The model under review builds one solid part; all positions refer to its coordinate system, in mm. A direction names the side the tool comes from. Round coordinates to 2 decimals unless told otherwise and drop trailing zeros. Order: outer loops, then holes, each group sorted by start corner. A loop starts at its lowest first (then second) coordinate and runs counter-clockwise, first axis right, second up. Notation, with made-up numbers: M -18.75,-24 L 0.25,-24 A23 ccw 0.25,-3 Z; hole C 28,84.25 d3. An arc over 180 degrees is marked long. One line per item, written item: value. Start each with the question number.
from build123d import *

# Parameters (mm, degrees)
SKETCH3_R          = 11
SKETCH3_R_2        = 10.2
CUT_EXTRUDE1_REACH = 197.895
SKETCH4_R          = 3.3
SKETCH5_R          = 3.3
CUT_EXTRUDE2_DEPTH = 196.894862351
CUT_EXTRUDE3_DEPTH = 196.894862351


with BuildPart() as part:
    # Sweep2: sweep along a path in Sketch1
    with BuildLine(Plane.XY) as sweep2_path:
        Line((108.839588828, 0), (92.239588828, 0))
        Line((92.239588828, 0), (-92.239588828, 0))
        ThreePointArc((-92.239588828, 0), (-124.360019313, -10.591729527), (-143.88004565, -38.211927945))
        Line((-143.88004565, -38.211927945), (-154.760411172, -73.8))
        Line((-154.760411172, -73.8), (-160.324709574, -92))
    # Sketch3 → Sweep2 (sweep)
    with BuildSketch(Plane(origin=(92.239588828, 0, 0), x_dir=(0, 0, -1), z_dir=(1, 0, 0))):
        Circle(SKETCH3_R)
        Circle(SKETCH3_R_2, mode=Mode.SUBTRACT)
    sweep(path=sweep2_path.line)

    # Sketch4 → Cut-Extrude1 (cut, up to next)
    with BuildSketch(Plane.XY, mode=Mode.PRIVATE) as cut_extrude1_sk1:
        with Locations(Location((-154.760411172, -73.8, 0), (0, 0, 163))):
            Circle(SKETCH4_R)
    cut_extrude1_tool1 = extrude(cut_extrude1_sk1.sketch, amount=CUT_EXTRUDE1_REACH, mode=Mode.PRIVATE) & part.part
    # Sketch4 → Cut-Extrude1 (cut, up to next)
    with BuildSketch(Plane.XY, mode=Mode.PRIVATE) as cut_extrude1_sk2:
        with BuildLine():
            Line((108.839588828, 2.555545653), (108.839588828, -2.555545653))
            Line((108.839588828, -2.555545653), (105.639588828, -2.555545653))
            ThreePointArc((105.639588828, -2.555545653), (104.225375266, -1.969759216), (103.639588828, -0.555545653))
            Line((103.639588828, -0.555545653), (103.639588828, 0.555545653))
            ThreePointArc((103.639588828, 0.555545653), (104.225375266, 1.969759216), (105.639588828, 2.555545653))
            Line((105.639588828, 2.555545653), (108.839588828, 2.555545653))
        make_face()
    cut_extrude1_tool2 = extrude(cut_extrude1_sk2.sketch, amount=CUT_EXTRUDE1_REACH, mode=Mode.PRIVATE) & part.part
    # Sketch4 → Cut-Extrude1 (cut, up to next)
    with BuildSketch(Plane.XY, mode=Mode.PRIVATE) as cut_extrude1_sk3:
        with BuildLine():
            Line((90.239588828, -5.5), (94.239588828, -5.5))
            ThreePointArc((94.239588828, -5.5), (95.653802391, -4.914213562), (96.239588828, -3.5))
            Line((96.239588828, -3.5), (96.239588828, 3.5))
            ThreePointArc((96.239588828, 3.5), (95.653802391, 4.914213562), (94.239588828, 5.5))
            Line((94.239588828, 5.5), (90.239588828, 5.5))
            ThreePointArc((90.239588828, 5.5), (88.825375266, 4.914213562), (88.239588828, 3.5))
            Line((88.239588828, 3.5), (88.239588828, -3.5))
            ThreePointArc((88.239588828, -3.5), (88.825375266, -4.914213562), (90.239588828, -5.5))
        make_face()
    cut_extrude1_tool3 = extrude(cut_extrude1_sk3.sketch, amount=CUT_EXTRUDE1_REACH, mode=Mode.PRIVATE) & part.part
    add(cut_extrude1_tool1.solids().sort_by_distance((-154.760411, -73.8, 0))[0], mode=Mode.SUBTRACT)
    add(cut_extrude1_tool2.solids().sort_by_distance((106.388287, 0, 0))[0], mode=Mode.SUBTRACT)
    add(cut_extrude1_tool3.solids().sort_by_distance((92.239589, 0, 0))[0], mode=Mode.SUBTRACT)

    # Sketch5 → Cut-Extrude2 (cut, through all)
    with BuildSketch(Plane.XY):
        with Locations(Location((-154.760411172, -73.8, 0), (0, 0, 163))):
            Circle(SKETCH5_R)
    extrude(amount=-CUT_EXTRUDE2_DEPTH, mode=Mode.SUBTRACT)

    # Sketch6 → Cut-Extrude3 (cut, through all)
    with BuildSketch(Plane.XY):
        with BuildLine():
            Line((108.839588828, 2.555545653), (105.639588828, 2.555545653))
            ThreePointArc((105.639588828, 2.555545653), (104.225375266, 1.969759216), (103.639588828, 0.555545653))
            Line((103.639588828, 0.555545653), (103.639588828, -0.555545653))
            ThreePointArc((103.639588828, -0.555545653), (104.225375266, -1.969759216), (105.639588828, -2.555545653))
            Line((105.639588828, -2.555545653), (108.839588828, -2.555545653))
            Line((108.839588828, -2.555545653), (108.839588828, 2.555545653))
        make_face()
    extrude(amount=-CUT_EXTRUDE3_DEPTH, mode=Mode.SUBTRACT)


solid = part.part
Item 1: The part is to be moulded in two halves that separate along Y. For faces 3 (the flat face through (108.84, -10.6, 0)), 4 (the flat face through (-154.14, -93.89, 8.1)), 5 (the cylindrical face through (-151.65, -74.9, -10.32)), 6 (the cylindrical face through (6.89, 10.74, 2.38)), say which applies: pulls with the +Y half, pulls with the -Y half, needs draft (parallel to the pull), parting line crosses it, or undercut.
Item 2: Clearance check with flat-ended pins moving along their axes: P1, Ø0.9, axis at x = 108, z = -10, coming from the +Y side; P2, Ø12, axis at x = -108, z = -2.5, coming from the -Y side; P3, Ø12, axis at y = -72.5, z = 3, coming from the +X side; P4, Ø6, axis at x = -154.76, y = -73.8, coming from the -Z side. State where each tip first meets the part, or that it passes through.
Item 3: Consider section A-A, the plane z = -0.25. Give the boundary of the cut face in (x, y).
Item 4: Wall thickness on L1, parallel to Y at x = -23, z = -0.25; L2, parallel to Y at x = -78, z = -6.5; L3, parallel to X at y = -76.5, z = 2.75: over which ranges is each line inside the solid? List them lowest first.
Item 5: Machinability: for faces 1 (the cylindrical face through (-151.65, -74.9, 10.32)), 2 (the cylindrical face through (6.892, 9.049, -4.707)), which of the approach directions +Z, -Z, +X, -X, +Y, -Y give a long, thin tool a straight path to every point of the face, cutting with its end or side? Answer none if there is none.
Item 6: Consider section B-B, the plane x = 76.5. Give the boundary of the cut face in (y, z), then the cut area to 3 significant figures.
Computed:
1. face 3: needs draft
1. face 4: pulls with the -Y half
1. face 5: undercut
1. face 6: parting line crosses it
2. P1: stops at y = 5.46
2. P2: stops at y = -16.75
2. P3: stops at x = -141.18
2. P4: passes through
3. outline: M -170.84,-88.78 L -170.08,-89.02 L -153.63,-35.23 A64.2 cw -92.24,10.2 L 108.84,10.2 L 108.84,11 L -92.24,11 A65 ccw -154.4,-35 Z; M -150.57,-94.98 L -149.81,-95.22 L -133.36,-41.43 A43 cw -92.24,-11 L 108.84,-11 L 108.84,-10.2 L -92.24,-10.2 A43.8 ccw -134.13,-41.19 Z
4. L1: y = -11 to -10.2, 10.2 to 11
4. L2: y = -8.87 to -7.86, 7.86 to 8.87
4. L3: x = -166.72 to -165.86, -145.31 to -144.45
5. face 1: +Z, -Z
5. face 2: +X
6. outline: C 0,0 d22; hole C 0,0 d20.4
6. area: 53.3 mm^2
